The model under review builds one solid part; all positions refer to its coordinate system, in mm. Face numbers are marked on the shaded views. A direction names the side the tool comes from. Round coordinates to 2 decimals unless told otherwise and drop trailing zeros. Write each loop counter-clockwise with the first axis right and the second up, starting at its lowest first coordinate (ties: lowest second). Pieces come first, ordered by that corner, then holes. Notation, with made-up numbers: (62.25, 35.5) -> (98.25, 35.5) arc R35 cw to (98.25, 71.5) -> close; hole circle Ø8 at (38, 7.5). An arc over 180 degrees is marked (long way). Use CSV: the item, a comma, the result in double quotes. Start each with the question number.
1) Take a section at A-A, the plane y = 0. Give the boundary of the cut face in (x, z).
2) For pin 1 Ø5 at (y, z) = (21.5, -346.5) entering from +X; pin 2 Ø10 at (y, z) = (27, -88) entering from +X; pin 3 Ø1 at (x, z) = (20.5, 276) entering from -Y, all flat-tipped, find the tip position at first contact; note any pin that passes through.
3) Machinability: for the marked faces 1, 2 and 3, which of the approach directions +Z, -Z, +X, -X, +Y, -Y give a long, thin tool a straight path to every point of the face, cutting with its end or side? Answer none if there is none.
4) Wall thickness on probe 1 along X at (y, z) = (-2, 282.5); probe 2 along X at (y, z) = (-1, 731.5); probe 3 along Y at (x, z) = (26, -669): over which ranges is each line inside the solid? List them lowest first. Write a range as [from, to].
5) Take a section at C-C, the plane z = -429.5. Give the boundary of the cut face in (x, y).
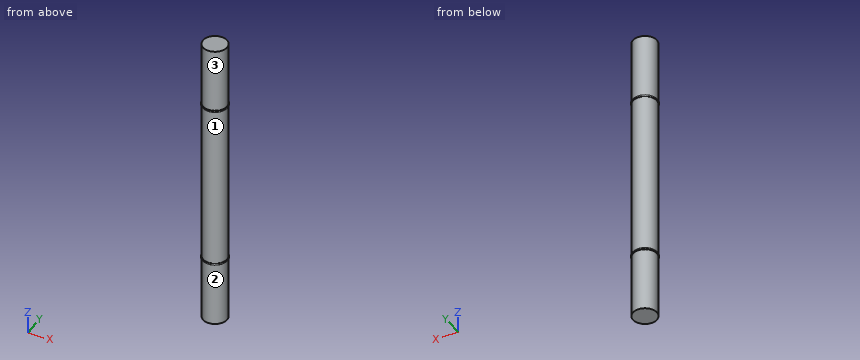
from build123d import *

# Parameters (mm, degrees)
F0_R          = 72.778
F1_DEPTH      = 900
F1_DEPTH_BACK = 900
F3_R          = 75
F3_R_2        = 72.778
F4_DEPTH      = 10


# Not quite as in the source:
# - a pattern or mirror of a feature is missing from the dataset's text; its kind, count and spacing are read off the source's solid


with BuildPart() as f1:
    # F0 (on Top) → F1 (new body, two sides)
    with BuildSketch(Plane.XY) as f1_sk:
        Circle(F0_R)
    extrude(amount=F1_DEPTH)
    extrude(f1_sk.sketch, amount=-F1_DEPTH_BACK)

    # F3 (on offset) → F4 (join)
    with BuildSketch(Plane.XY.offset(500)):
        Circle(F3_R)
        Circle(F3_R_2, mode=Mode.SUBTRACT)
    f4 = extrude(amount=F4_DEPTH)

    # F4_copies: F4 across plane
    add(f4.mirror(Plane(origin=(0, 0, 0), x_dir=(-1, 0, 0), z_dir=(0, 0, -1))))


solid = f1.part
Values found:
1,outline,"(-75, -510) -> (-72.78, -510) -> (-72.78, -900) -> (72.78, -900) -> (72.78, -510) -> (75, -510) -> (75, -500) -> (72.78, -500) -> (72.78, 500) -> (75, 500) -> (75, 510) -> (72.78, 510) -> (72.78, 900) -> (-72.78, 900) -> (-72.78, 510) -> (-75, 510) -> (-75, 500) -> (-72.78, 500) -> (-72.78, -500) -> (-75, -500) -> close"
2,pin 1,"x = 70.25"
2,pin 2,"x = 69.37"
2,pin 3,"y = -69.98"
3,face 1,"none"
3,face 2,"-Z"
3,face 3,"+Z"
4,probe 1,"[-72.75, 72.75]"
4,probe 2,"[-72.77, 72.77]"
4,probe 3,"[-67.98, 67.98]"
5,outline,"circle Ø145.56 at (0, 0)"
